Part model, mm, in its own coordinate system. A direction names the side the tool comes from. Round coordinates to 2 decimals unless told otherwise and drop trailing zeros. Order: outer loops, then holes, each group sorted by start corner. A loop starts at its lowest first (then second) coordinate and runs counter-clockwise, first axis right, second up. Notation, with made-up numbers: M -24.5,33.25 L 10.5,33.25 A16 ccw 10.5,51.25 Z; hole C 55,78.5 d11. An arc over 180 degrees is marked long. Write each question's results on one line, items separated by ' | '. Start each with the question number.
1. Band-saw the part on A-A, the plane y = 12.5. List the corners of the cut face in (x, z).
2. Drop flat-ended pins along their axis: pin 1 Ø0.8 at (x, z) = (10.5, 14.5) entering from +Y; pin 2 Ø0.5 at (y, z) = (11.5, 14.5) entering from +X; pin 3 Ø12 at (x, y) = (14.5, 37) entering from +Z. Give the stop position or say it passes through.
3. Probe L1, parallel to Z at x = 17.5, y = 5. List the from-to ranges inside material, lowest first. Write a range as [from, to].
4. Band-saw the part on B-B, the plane x = 5. List the corners of the cut face in (y, z), then the cut area to 3 significant figures.
5. Two-plate mould, pull along Y, no slides. Class faces 5 (the face through (12, 21, 14.5)), 6 (the face through (21.6, 14, 14.5)), 7 (the face through (22.6, 23, 14.5)): +Y half, -Y half, draft (parallel to the pull), parting line (faces both ways), or undercut.
6. Which spindle directions (+Z, -Z, +X, -X, +Y, -Y) get a long thin tool onto all of the face, cutting with end or side? Do faces 1 (the face through (32.6, 19, 14.5)), 2 (the face through (23.2, 21, 14.5)), 3 (the face through (19.6, 14, 14.5)), 4 (the face through (28, 21, 14.5)). Say none if no direction does.
```python
from build123d import *

# Parameters (mm, degrees)
BOSS_EXTRUDE1_DEPTH = 14
SKETCH2_W           = 7
SKETCH2_H           = 5
SKETCH2_W_2         = 5
BOSS_EXTRUDE2_DEPTH = 0.5
SKETCH3_W           = 1.2
SKETCH3_H           = 4
BOSS_EXTRUDE3_DEPTH = 1
SKETCH4_W           = 2
SKETCH4_H           = 5
BOSS_EXTRUDE4_DEPTH = 3


with BuildPart() as part:
    # Sketch1 → Boss-Extrude1 (new body)
    with BuildSketch(Plane.XY):
        with BuildLine():
            Line((1, 0), (44, 0))
            ThreePointArc((44, 0), (44.707106781, 0.292893219), (45, 1))
            Line((45, 1), (45, 41))
            ThreePointArc((45, 41), (44.707106781, 41.707106781), (44, 42))
            Line((44, 42), (1, 42))
            ThreePointArc((1, 42), (0.292893219, 41.707106781), (0, 41))
            Line((0, 41), (0, 1))
            ThreePointArc((0, 1), (0.292893219, 0.292893219), (1, 0))
        make_face()
    extrude(amount=BOSS_EXTRUDE1_DEPTH)

    # Sketch2 → Boss-Extrude2 (add)
    with BuildSketch(Plane.XY.offset(14)):
        with Locations((18.5, 27.5)):
            Rectangle(SKETCH2_W, SKETCH2_H)
        with Locations((27.5, 27.5)):
            Rectangle(SKETCH2_W_2, SKETCH2_H)
    extrude(amount=BOSS_EXTRUDE2_DEPTH)

    # Sketch3 → Boss-Extrude3 (add)
    with BuildSketch(Plane.XY.offset(14)):
        with Locations((10.6, 21)):
            Rectangle(SKETCH3_W, SKETCH3_H)
        with Locations((12.6, 21)):
            Rectangle(SKETCH3_W, SKETCH3_H)
        with Locations((14.6, 21)):
            Rectangle(SKETCH3_W, SKETCH3_H)
        with Locations((16.6, 21)):
            Rectangle(SKETCH3_W, SKETCH3_H)
        with Locations((18.6, 21)):
            Rectangle(SKETCH3_W, SKETCH3_H)
        with Locations((20.6, 21)):
            Rectangle(SKETCH3_W, SKETCH3_H)
        with Locations((22.6, 21)):
            Rectangle(SKETCH3_W, SKETCH3_H)
        with Locations((24.6, 21)):
            Rectangle(SKETCH3_W, SKETCH3_H)
        with Locations((26.6, 21)):
            Rectangle(SKETCH3_W, SKETCH3_H)
        with Locations((28.6, 21)):
            Rectangle(SKETCH3_W, SKETCH3_H)
        with Locations((30.6, 21)):
            Rectangle(SKETCH3_W, SKETCH3_H)
        with Locations((32.6, 21)):
            Rectangle(SKETCH3_W, SKETCH3_H)
        with Locations((19.6, 12)):
            Rectangle(SKETCH3_W, SKETCH3_H)
        with Locations((17.6, 12)):
            Rectangle(SKETCH3_W, SKETCH3_H)
        with Locations((21.6, 12)):
            Rectangle(SKETCH3_W, SKETCH3_H)
        with Locations((23.6, 12)):
            Rectangle(SKETCH3_W, SKETCH3_H)
        with Locations((25.6, 12)):
            Rectangle(SKETCH3_W, SKETCH3_H)
        with Locations((27.6, 12)):
            Rectangle(SKETCH3_W, SKETCH3_H)
    extrude(amount=BOSS_EXTRUDE3_DEPTH)

    # Sketch4 → Boss-Extrude4 (add)
    with BuildSketch(Plane.XY.offset(14)):
        with Locations((12, 27.5)):
            Rectangle(SKETCH4_W, SKETCH4_H)
    extrude(amount=BOSS_EXTRUDE4_DEPTH)


solid = part.part
```
Solution:
1) outline: M 0,0 L 45,0 L 45,14 L 28.2,14 L 28.2,15 L 27,15 L 27,14 L 26.2,14 L 26.2,15 L 25,15 L 25,14 L 24.2,14 L 24.2,15 L 23,15 L 23,14 L 22.2,14 L 22.2,15 L 21,15 L 21,14 L 20.2,14 L 20.2,15 L 19,15 L 19,14 L 18.2,14 L 18.2,15 L 17,15 L 17,14 L 0,14 Z
2) pin 1: y = 23 | pin 2: x = 28.2 | pin 3: z = 14
3) L1: [0, 14]
4) outline: M 0,0 L 42,0 L 42,14 L 0,14 Z | area: 588 mm^2
5) face 5: draft | face 6: undercut | face 7: +Y half
6) face 1: +Z, +X, -X, -Y | face 2: +Z, +Y | face 3: +Z, +X, -X | face 4: +Z
